Read the model definition and answer for the solid it produces. Units are mm, in the model's axes. Coordinates: 2 decimals unless noted, no trailing zeros. Write each loop counter-clockwise with the first axis right and the second up, starting at its lowest first coordinate (ties: lowest second). Pieces come first, ordered by that corner, then holes.
(1) The part is cut by section A-A, the plane z = 7. Determine the outline of the cut face in (x, y).
(2) Given pin 1 (1.5 mm diameter, centred on x = -1.5, z = 10.5, fed in from +Y); pin 2 (3 mm diameter, centred on x = -2, y = 3.5, fed in from -Z); pin 3 (5 mm diameter, centred on y = -4, z = 12.5, fed in from -X); pin 4 (2 mm diameter, centred on y = 3.5, z = 8, fed in from +X), each flat-ended and moving along its own axis, determine where each tip first touches the part or whether it passes through.
(3) Straight lines are drawn through the part: line 1 along Y through (x, z) = (0, 27.6); line 2 along X through (y, z) = (-0.25, 16); line 3 along X through (y, z) = (2.5, 27.25). For each, find the intervals that lie inside material, in ascending order.
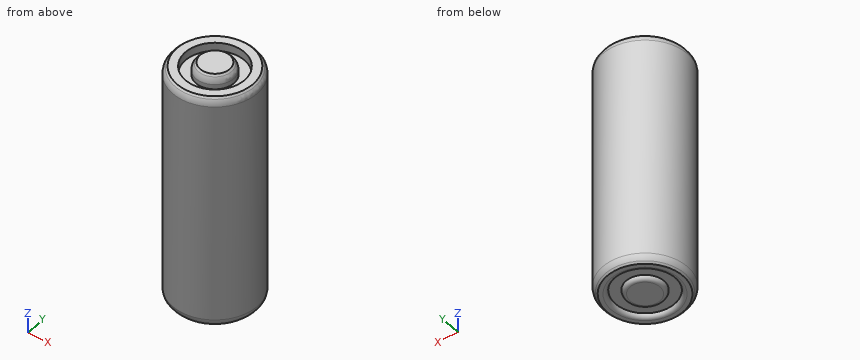
```python
from build123d import *

# Parameters (mm, degrees)
SKETCH_R        = 5
PAD_DEPTH       = 28
CHAMFER_SIZE    = 0.5
CHAMFER001_SIZE = 0.5
SKETCH001_R     = 3.5
POCKET_DEPTH    = 1
FILLET_R        = 1
FILLET001_R     = 1
SKETCH002_R     = 2.25
PAD001_DEPTH    = 1.5
CHAMFER002_SIZE = 0.5
FILLET002_R     = 1
SKETCH003_R     = 3.5
POCKET001_DEPTH = 0.5
SKETCH004_R     = 2.25
POCKET002_DEPTH = 1
SKETCH005_R     = 2.25
PAD002_DEPTH    = 1
PAD003_DEPTH    = 1.5
FILLET003_R     = 0.49
FILLET004_R     = 0.49


with BuildPart() as part:
    # Sketch → Pad (new body)
    with BuildSketch(Plane.XY):
        Circle(SKETCH_R)
    extrude(amount=PAD_DEPTH)

    # Chamfer
    chamfer_edges = [part.edges().sort_by_distance(p)[0] for p in [
        (-5, 0, 0),
    ]]
    chamfer(chamfer_edges, length=CHAMFER_SIZE)

    # Chamfer001
    chamfer001_edges = [part.edges().sort_by_distance(p)[0] for p in [
        (-5, 0, 28),
    ]]
    chamfer(chamfer001_edges, length=CHAMFER001_SIZE)

    # Sketch001 (on Face4 of Chamfer001) → Pocket (cut)
    with BuildSketch(Plane.XY.offset(28)):
        Circle(SKETCH001_R)
    extrude(amount=-POCKET_DEPTH, mode=Mode.SUBTRACT)

    # Fillet
    fillet_edges = [part.edges().sort_by_distance(p)[0] for p in [
        (-5, 0, 27.5),
    ]]
    fillet(fillet_edges, radius=FILLET_R)

    # Fillet001
    fillet001_edges = [part.edges().sort_by_distance(p)[0] for p in [
        (-5, 0, 0.5),
    ]]
    fillet(fillet001_edges, radius=FILLET001_R)

    # Sketch002 (on Face9 of Fillet001) → Pad001 (join)
    with BuildSketch(Plane.XY.offset(27)):
        Circle(SKETCH002_R)
    extrude(amount=PAD001_DEPTH)

    # Chamfer002
    chamfer002_edges = [part.edges().sort_by_distance(p)[0] for p in [
        (-2.25, 0, 28.5),
    ]]
    chamfer(chamfer002_edges, length=CHAMFER002_SIZE)

    # Fillet002
    fillet002_edges = [part.edges().sort_by_distance(p)[0] for p in [
        (-2.25, 0, 28),
    ]]
    fillet(fillet002_edges, radius=FILLET002_R)

    # Sketch003 (on Face6 of Pad001) → Pocket001 (cut)
    with BuildSketch(Plane(origin=(0, 0, 0), x_dir=(1, 0, 0), z_dir=(0, 0, -1))):
        Circle(SKETCH003_R)
    extrude(amount=-POCKET001_DEPTH, mode=Mode.SUBTRACT)

    # Sketch004 (on Face15 of Pocket001) → Pocket002 (cut)
    with BuildSketch(Plane(origin=(0, 0, 0.5), x_dir=(1, 0, 0), z_dir=(0, 0, -1))):
        Circle(SKETCH004_R)
    extrude(amount=-POCKET002_DEPTH, mode=Mode.SUBTRACT)

    # Sketch005 (on Face17 of Pocket002) → Pad002 (join)
    with BuildSketch(Plane(origin=(0, 0, 1.5), x_dir=(1, 0, 0), z_dir=(0, 0, -1))):
        Circle(SKETCH005_R)
    extrude(amount=PAD002_DEPTH)

    # Sketch005 (on Face17 of Pocket002) → Pad003 (join)
    with BuildSketch(Plane(origin=(0, 0, 1.5), x_dir=(1, 0, 0), z_dir=(0, 0, -1))):
        Circle(SKETCH005_R)
    extrude(amount=PAD003_DEPTH)

    # Fillet003
    fillet003_edges = [part.edges().sort_by_distance(p)[0] for p in [
        (-2.25, 0, 0),
    ]]
    fillet(fillet003_edges, radius=FILLET003_R)

    # Fillet004
    fillet004_edges = [part.edges().sort_by_distance(p)[0] for p in [
        (-3.5, 0, 0),
    ]]
    fillet(fillet004_edges, radius=FILLET004_R)


solid = part.part
```
Computed:
1. outline: circle Ø10 at (0, 0)
2. pin 1: stops at y = 4.94
2. pin 2: stops at z = 0
2. pin 3: stops at x = -4.77
2. pin 4: stops at x = 4.33
3. line 1: y = -4.86 to -3.5, -2.25 to 2.25, 3.5 to 4.86
3. line 2: x = -4.99 to 4.99
3. line 3: x = -4.31 to -2.45, 2.45 to 4.31
